Work out the finished part from the listing and answer in its coordinate system (mm). A direction names the side the tool comes from. Round coordinates to 2 decimals unless told otherwise and drop trailing zeros. Write each loop counter-clockwise with the first axis right and the second up, starting at its lowest first coordinate (ties: lowest second). Pieces come first, ordered by that corner, then holes. Notation, with made-up numbers: (23, 84) -> (64, 84) arc R13 ccw to (64, 109) -> close; hole circle Ø7 at (76.5, 37.25). An arc over 180 degrees is marked (long way). One line per item, written item: value.
```python
from build123d import *

# Parameters (mm, degrees)
F1_DEPTH = 20
F2_W     = 20
F2_H     = 15
F3_DEPTH = 50.001
F4_W     = 10
F4_H     = 22.5
F4_H_2   = 5
F5_DEPTH = 28


with BuildPart() as f1:
    # F0 (on Right) → F1 (new body, symmetric)
    with BuildSketch(Plane.YZ):
        Polygon((-25, 15), (0, 15), (0, 50), (-2.5, 50), align=None)
        Polygon((25, -15), (25, 15), (0, 15), (-25, 15), (-25, -15), align=None)
        Polygon((0, 15), (25, 15), (2.5, 50), (0, 50), align=None)
    extrude(amount=F1_DEPTH, both=True)

    # F2 (on face) → F3 (cut, through all)
    with BuildSketch(Plane.XZ.offset(25)):
        with Locations((-10, -7.5)):
            Rectangle(F2_W, F2_H)
    extrude(amount=-F3_DEPTH, mode=Mode.SUBTRACT)

    # F4 (on face) → F5 (cut)
    with BuildSketch(Plane.XY.offset(50)):
        with Locations((0, -13.75)):
            Rectangle(F4_W, F4_H)
        Rectangle(F4_W, F4_H_2)
        with Locations((0, 13.75)):
            Rectangle(F4_W, F4_H)
    extrude(amount=-F5_DEPTH, mode=Mode.SUBTRACT)


solid = f1.part
```
(1) Find section B-B on x = -1. Give the vertices of the cut face in (y, z), plus the area to 3 significant figures.
Reported:
outline: (-25, 0) -> (25, 0) -> (25, 15) -> (20.5, 22) -> (-20.5, 22) -> (-25, 15) -> close
area: 1,070 mm2
(2) Find section C-C on y = 8.5. Give the vertices of the cut face in (x, z).
Reported:
outline: (-20, 0) -> (0, 0) -> (0, -15) -> (20, -15) -> (20, 40.67) -> (5, 40.67) -> (5, 22) -> (-5, 22) -> (-5, 40.67) -> (-20, 40.67) -> close
(3) Flat-ended cylindrical pins translate along their axes: pin 1 Ø1.5 at (x, y) = (-2.5, 13) entering from -Z; pin 2 Ø4.5 at (y, z) = (-12, -6) entering from -X; pin 3 Ø3 at (x, z) = (14.5, 20) entering from -Y. Find the tip coordinate at first contact, or state that the pin passes through.
Reported:
pin 1: stops at z = 0
pin 2: stops at x = 0
pin 3: stops at y = -22.75
(4) Find section D-D on x = 17. Give the vertices of the cut face in (y, z), plus the area to 3 significant figures.
Reported:
outline: (-25, -15) -> (25, -15) -> (25, 15) -> (2.5, 50) -> (-2.5, 50) -> (-25, 15) -> close
area: 2,460 mm2
(5) A tool of negligible diameter and unlimited length cuts with its end or side. For faces 1 (the face through (0, 0, -8)), 2 (the face through (5, 25, 3)), 3 (the face through (5, 0, 33)), from which of +Z, -Z, +X, -X, +Y, -Y can it reach the whole face along a straight path? Write none if from no direction.
Reported:
face 1: -Z, -X, +Y, -Y
face 2: +Z, -Z, +X, -X, +Y
face 3: +Z, +Y, -Y
(6) Find section A-A on z = 28. Give the vertices of the cut face in (x, y), plus the area to 3 significant figures.
Reported:
outline: (-20, -16.64) -> (-5, -16.64) -> (-5, 16.64) -> (-20, 16.64) -> close; (5, -16.64) -> (20, -16.64) -> (20, 16.64) -> (5, 16.64) -> close
area: 999 mm2
(7) Consider probe 1 along X at (y, z) = (-17.5, 26); probe 2 along Z at (x, y) = (3, -8); probe 3 along Z at (x, y) = (-7.5, -0.5). Determine where each line is inside the solid, lowest interval first.
Reported:
probe 1: x = -20 to -5, 5 to 20
probe 2: z = -15 to 22
probe 3: z = 0 to 50
